The listing builds one solid part. Answer for the finished solid, in the listing's coordinates (mm). A direction names the side the tool comes from. Coordinates: 2 decimals unless noted, no trailing zeros. Loops run counter-clockwise (first coordinate to the right, second up) from the corner with the lowest first, then second, coordinate; pieces in that order, holes last. Notation, with made-up numbers: (56.25, 87) - (97.25, 87) arc R8 cw to (97.25, 93) - close; hole circle Ø8 at (-22.5, 37). An arc over 180 degrees is marked (long way). Return JSON: item names as keys, results as strings. Group by question number.
1. Each of these flat-tipped pins is pushed along its axis until it touches: P1, Ø2.5, axis at x = -8, z = 13, coming from the +Y side; P2, Ø4, axis at x = 14, y = 39, coming from the +Z side; P3, Ø2, axis at x = 0.5, y = 22.5, coming from the -Z side. Where does it stop, or does it pass through?
2. Section C-C (z = 0) is taken. Write down the section's boundary in (x, y), and give its area (3 significant figures).
3. Find the intervals of material crossed by line 1 along X through (y, z) = (46.5, 0); line 2 along Z through (x, y) = (-7, 47); line 3 along Y through (x, z) = (0, -6), in increasing order.
4. The mould has two halves that part along X. Classify faces 4 (the face through (0, 53, 0)), 5 (the face through (-15, 43, 0)), 6 (the face through (-7.086, 42.86, 17.089)): pulls with the +X half, pulls with the -X half, needs draft (parallel to the pull), parting line crosses it, or undercut.
5. Which of the six approach directions +Z, -Z, +X, -X, +Y, -Y give full straight-line access (tool end or side, diameter ignored) to faces 1 (the face through (-16.4, 33, 5.4)), 2 (the face through (0, 64, -9.5)), 3 (the face through (-8, 43, 13))?
6. Section D-D (x = -12) is taken. Write down the section's boundary in (y, z).
7. Section A-A (x = 0) is taken. Write down the section's boundary in (y, z), and give its area (3 significant figures).
8. Section B-B (y = 70) is taken. Write down the section's boundary in (x, z), and give its area (3 significant figures).
```python
from build123d import *

# Parameters (mm, degrees)
SKETCH1_R           = 17
BOSS_EXTRUDE1_DEPTH = 33
SKETCH2_R           = 18.5
BOSS_EXTRUDE2_DEPTH = 20
SKETCH3_R           = 6
BOSS_EXTRUDE3_DEPTH = 5
SKETCH4_R           = 3
BOSS_EXTRUDE4_DEPTH = 15
CUT_EXTRUDE1_START  = -14
CUT_EXTRUDE1_DEPTH  = 14
SKETCH6_R           = 1.5
CUT_EXTRUDE2_DEPTH  = 10
SKETCH7_R           = 1.6
CUT_EXTRUDE3_DEPTH  = 10


with BuildPart() as part:
    # Sketch1 → Boss-Extrude1 (new body)
    with BuildSketch(Plane(origin=(0, 0, 0), x_dir=(1, 0, 0), z_dir=(0, 1, 0))):
        with Locations(Location((0, 0, 0), (0, 0, 270))):
            Circle(SKETCH1_R)
    extrude(amount=BOSS_EXTRUDE1_DEPTH)

    # Sketch2 → Boss-Extrude2 (add)
    with BuildSketch(Plane(origin=(0, 33, 0), x_dir=(1, 0, 0), z_dir=(0, 1, 0))):
        with Locations(Location((0, 0, 0), (0, 0, 270))):
            Circle(SKETCH2_R)
    extrude(amount=BOSS_EXTRUDE2_DEPTH)

    # Sketch3 → Boss-Extrude3 (add)
    with BuildSketch(Plane(origin=(0, 53, 0), x_dir=(1, 0, 0), z_dir=(0, 1, 0))):
        with Locations(Location((0, 7, 0), (0, 0, 270))):
            Circle(SKETCH3_R)
    extrude(amount=BOSS_EXTRUDE3_DEPTH)

    # Sketch4 → Boss-Extrude4 (add)
    with BuildSketch(Plane(origin=(0, 58, 0), x_dir=(1, 0, 0), z_dir=(0, 1, 0))):
        with Locations(Location((0, 7, 0), (0, 0, 270))):
            Circle(SKETCH4_R)
    extrude(amount=BOSS_EXTRUDE4_DEPTH)

    # Sketch5 → Cut-Extrude1 (cut)
    with BuildSketch(Plane(origin=(0, 73, 0), x_dir=(1, 0, 0), z_dir=(0, 1, 0)).offset(CUT_EXTRUDE1_START)):
        with BuildLine():
            Line((-1.658312395, 9.5), (1.658312395, 9.5))
            ThreePointArc((1.658312395, 9.5), (0, 10), (-1.658312395, 9.5))
        make_face()
    extrude(amount=CUT_EXTRUDE1_DEPTH, mode=Mode.SUBTRACT)

    # Sketch6 → Cut-Extrude2 (cut)
    with BuildSketch(Plane(origin=(0, 53, 0), x_dir=(1, 0, 0), z_dir=(0, 1, 0))):
        with Locations(Location((15.5, 0, 0), (0, 0, 270))):
            Circle(SKETCH6_R)
        with Locations(Location((-15.5, 0, 0), (0, 0, 270))):
            Circle(SKETCH6_R)
        with Locations(Location((-7.75, -13.423393759, 0), (0, 0, 270))):
            Circle(SKETCH6_R)
        with Locations(Location((7.75, -13.423393759, 0), (0, 0, 270))):
            Circle(SKETCH6_R)
        with Locations(Location((-7.75, 13.423393759, 0), (0, 0, 270))):
            Circle(SKETCH6_R)
        with Locations(Location((7.75, 13.423393759, 0), (0, 0, 270))):
            Circle(SKETCH6_R)
    extrude(amount=-CUT_EXTRUDE2_DEPTH, mode=Mode.SUBTRACT)

    # Sketch7 → Cut-Extrude3 (cut)
    with BuildSketch(Plane(origin=(0, 0, -9.5), x_dir=(-1, 0, 0), z_dir=(0, 0, -1))):
        with Locations((0, 70)):
            Circle(SKETCH7_R)
    extrude(amount=-CUT_EXTRUDE3_DEPTH, mode=Mode.SUBTRACT)


solid = part.part
```
The answers:
{
 "1": {"P1": "stops at y = 53", "P2": "stops at z = 14.08", "P3": "stops at z = -17"},
 "2": {"outline": "(-18.5, 33) - (-17, 33) - (-17, 0) - (17, 0) - (17, 33) - (18.5, 33) - (18.5, 53) - (17, 53) - (17, 43) - (14, 43) - (14, 53) - (-14, 53) - (-14, 43) - (-17, 43) - (-17, 53) - (-18.5, 53) - close", "area": "1,800 mm2"},
 "3": {"line 1": "x = -18.5 to -17, -14 to 14, 17 to 18.5", "line 2": "z = -17.12 to -14.72, -12.12 to 12.12, 14.72 to 17.12", "line 3": "y = 0 to 68.4, 71.6 to 73"},
 "4": {"face 4": "needs draft", "face 5": "undercut", "face 6": "parting line crosses it"},
 "5": {"face 1": "-Y", "face 2": "-Z, +X, -X, +Y", "face 3": "+Y"},
 "6": {"outline": "(0, -12.04) - (33, -12.04) - (33, -14.08) - (53, -14.08) - (53, 14.08) - (33, 14.08) - (33, 12.04) - (0, 12.04) - close"},
 "7": {"outline": "(0, -17) - (33, -17) - (33, -18.5) - (53, -18.5) - (53, -13) - (58, -13) - (58, -10) - (59, -10) - (59, -9.5) - (68.4, -9.5) - (68.4, -4) - (58, -4) - (58, -1) - (53, -1) - (53, 18.5) - (33, 18.5) - (33, 17) - (0, 17) - close; (71.6, -9.5) - (73, -9.5) - (73, -4) - (71.6, -4) - close", "area": "1,990 mm2"},
 "8": {"outline": "(-1.66, -9.5) - (-1.6, -9.5) - (-1.6, -4.46) arc R3 ccw to start; (1.6, -9.5) - (1.66, -9.5) arc R3 ccw to (1.6, -4.46) - close", "area": "10.0 mm2"}
}
